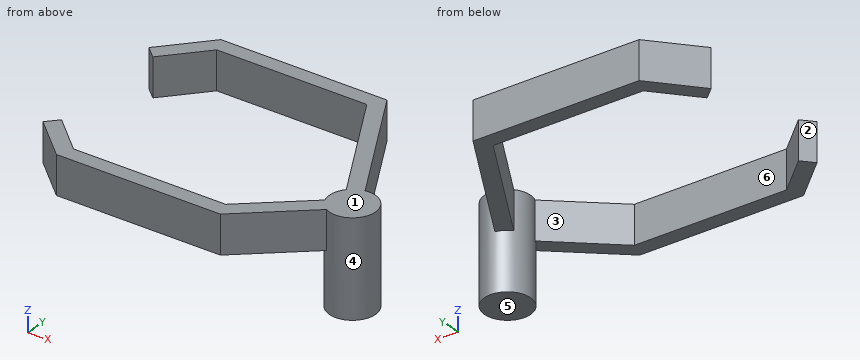
```python
from build123d import *

# Parameters (mm, degrees)
BOSS_EXTRUDE1_DEPTH = 10
SKETCH2_R           = 6
BOSS_EXTRUDE2_DEPTH = 25


with BuildPart() as part:
    # Sketch1 → Boss-Extrude1 (new body)
    with BuildSketch(Plane.XY):
        with BuildLine():
            ThreePointArc((-4.488845509, 3.981239254), (-2.90504438, 5.249830202), (-0.988958707, 5.917935508))
            Line((-0.988958707, 5.917935508), (-19.535932482, 39.434966685))
            Line((-19.535932482, 39.434966685), (-62.745195449, 39.434966685))
            Line((-62.745195449, 39.434966685), (-73.107309745, 27.816838535))
            Line((-73.107309745, 27.816838535), (-70.122128007, 25.154379147))
            Line((-70.122128007, 25.154379147), (-60.952955338, 35.434966685))
            Line((-60.952955338, 35.434966685), (-21.894070174, 35.434966685))
            Line((-21.894070174, 35.434966685), (-4.488845509, 3.981239254))
        make_face()
        with BuildLine():
            Line((2.535804531, -0.451815201), (-2.972059937, -5.212183777))
            ThreePointArc((-2.972059937, -5.212183777), (3.013937655, -5.188080552), (6, 0))
            ThreePointArc((6, 0), (3.877257262, 4.578960157), (-0.988958707, 5.917935508))
            Line((-0.988958707, 5.917935508), (2.535804531, -0.451815201))
        make_face()
        with BuildLine():
            ThreePointArc((-5.587664835, -2.185864062), (-4.539479574, -3.923407346), (-2.972059937, -5.212183777))
            Line((-2.972059937, -5.212183777), (2.535804531, -0.451815201))
            Line((2.535804531, -0.451815201), (-0.988958707, 5.917935508))
            ThreePointArc((-0.988958707, 5.917935508), (-2.90504438, 5.249830202), (-4.488845509, 3.981239254))
            Line((-4.488845509, 3.981239254), (-2.535804531, 0.451815201))
            Line((-2.535804531, 0.451815201), (-5.587664835, -2.185864062))
        make_face()
        with BuildLine():
            Line((-72.966168133, -10.42614814), (-62.627042774, -19.903679719))
            Line((-62.627042774, -19.903679719), (-19.970484994, -19.903679719))
            Line((-19.970484994, -19.903679719), (-2.972059937, -5.212183777))
            ThreePointArc((-2.972059937, -5.212183777), (-4.539479574, -3.923407346), (-5.587664835, -2.185864062))
            Line((-5.587664835, -2.185864062), (-21.459517662, -15.903679719))
            Line((-21.459517662, -15.903679719), (-61.071108012, -15.903679719))
            Line((-61.071108012, -15.903679719), (-70.263269619, -7.477531579))
            Line((-70.263269619, -7.477531579), (-72.966168133, -10.42614814))
        make_face()
    extrude(amount=BOSS_EXTRUDE1_DEPTH)

    # Sketch2 → Boss-Extrude2 (add)
    with BuildSketch(Plane.XY.offset(10)):
        Circle(SKETCH2_R)
    extrude(amount=-BOSS_EXTRUDE2_DEPTH)


solid = part.part
```
Verification items for the finished model (mm, model axes). Face numbers are marked on the shaded views. A direction names the side the tool comes from. Coordinates: 2 decimals unless noted, no trailing zeros. Loops run counter-clockwise (first coordinate to the right, second up) from the corner with the lowest first, then second, coordinate; pieces in that order, holes last. Notation, with made-up numbers: (79.5, -1) - (96.5, -1) arc R13 ccw to (96.5, 9) - close; hole circle Ø7 at (73, 24). An arc over 180 degrees is marked (long way). Put each result on its own line as item: value.
Item 1: Scan lines: line 1 along X through (y, z) = (0.5, -7.75); line 2 along Z through (x, y) = (-56.5, 35.5); line 3 along X through (y, z) = (-2, -11.25). Record each from-to range of solid material in increasing order.
Conclusion:
line 1: x = -5.98 to 5.98
line 2: z = 0 to 10
line 3: x = -5.66 to 5.66
Item 2: Section check B-B (y = 30.5). Enter the section's corners in (x, z), then the cut area to 3 significant figures.
Conclusion:
outline: (-70.71, 0) - (-65.35, 0) - (-65.35, 10) - (-70.71, 10) - close; (-19.16, 0) - (-14.59, 0) - (-14.59, 10) - (-19.16, 10) - close
area: 99.3 mm2
Item 3: Section check C-C (z = 8.25). Enter the section's corners in (x, y).
Conclusion:
outline: (-73.11, 27.82) - (-70.12, 25.15) - (-60.95, 35.43) - (-21.89, 35.43) - (-4.49, 3.98) arc R6 ccw to (-5.59, -2.19) - (-21.46, -15.9) - (-61.07, -15.9) - (-70.26, -7.48) - (-72.97, -10.43) - (-62.63, -19.9) - (-19.97, -19.9) - (-2.97, -5.21) arc R6 ccw (long way) to (-0.99, 5.92) - (-19.54, 39.43) - (-62.75, 39.43) - close
Item 4: Draft check along X on the marked faces 1, 2 and 3. Enter one of: pulls with the +X half, pulls with the -X half, needs draft (parallel to the pull), parting line crosses it, or undercut.
Conclusion:
face 1: needs draft
face 2: pulls with the -X half
face 3: undercut
Item 5: Section check D-D (z = -12.5). Enter the section's corners in (x, y), then the cut area to 3 significant figures.
Conclusion:
outline: circle Ø12 at (0, 0)
area: 113 mm2
Item 6: Section check A-A (x = -44). Enter the section's corners in (y, z), then the cut area to 3 significant figures.
Conclusion:
outline: (-19.9, 0) - (-15.9, 0) - (-15.9, 10) - (-19.9, 10) - close; (35.43, 0) - (39.43, 0) - (39.43, 10) - (35.43, 10) - close
area: 80.0 mm2
Item 7: Set-up check for the marked faces 4, 5 and 6: record each of +Z, -Z, +X, -X, +Y, -Y from which the full face is reachable in a straight line by a thin tool's end or side.
Conclusion:
face 4: -Z
face 5: -Z, +X, -X, +Y, -Y
face 6: +Z, -Z
Item 8: Gauge pin test, flat ends, axial feed: pin 1 Ø5.5 at (x, y) = (-22.5, -15) entering from -Z; pin 2 Ø10 at (y, z) = (7.5, -11) entering from +X; pin 3 Ø4 at (x, y) = (-13, -4.5) entering from -Z; pin 4 Ø3 at (y, z) = (3.5, -8.5) entering from +X. Record the tip position at first contact, or that the pin passes through.
Conclusion:
pin 1: stops at z = 0
pin 2: stops at x = 5.45
pin 3: passes through
pin 4: stops at x = 5.66
